Build history of the part. All positions in model axes, mm. Round coordinates to 2 decimals unless told otherwise and drop trailing zeros. Write each loop counter-clockwise with the first axis right and the second up, starting at its lowest first coordinate (ties: lowest second). Pieces come first, ordered by that corner, then holes. Notation, with made-up numbers: (37.25, -34) - (78.25, -34) arc R36 ccw to (78.25, 5) - close; hole circle Ø4 at (59, 35.25). An arc over 180 degrees is marked (long way). Answer as a JSON object with one key per item and string values. Group by question number.
Item 1: Probe line 1 (X direction, y = -0.25, z = 16); line 2 (X direction, y = 0.3, z = 15.25); line 3 (Z direction, x = 4, y = 0.05). List the from-to ranges inside material, lowest first. Write a range as from..to.
Item 2: Slice it at A-A, the plane y = -0.25. List the corners of the cut face in (x, z) (3 decimals).
Item 3: Slice it at D-D, the plane x = 6.75. List the corners of the cut face in (y, z) (3 decimals), then the cut area to 3 significant figures.
Item 4: Slice it at B-B, the plane z = 18.25. List the corners of the cut face in (x, y) (3 decimals), then the cut area to 3 significant figures.
Item 5: Slice it at C-C, the plane x = 10.25. List the corners of the cut face in (y, z) (3 decimals).
Solid Edge part; units mm, degrees
sketch "Sketch1" plane through (0, 0, 0) normal (0, -1, 0) x (1, 0, 0)
  line L0 (0, 0) -> (0, 5.75)
  line L1 (0, 11.5) -> (0, 5.75)
  line L2 (11.625, 21.5) -> (0, 11.5)
  line L3 (14.125, 21.5) -> (11.625, 21.5)
  line L4 (14.125, 21.5) -> (16.625, 21.5)
  line L5 (16.625, 21.5) -> (28.25, 11.5)
  line L6 (28.25, 0) -> (28.25, 11.5)
  line L7 (0, 0) -> (28.25, 0)
  circle A0 centre (14.125, 18.25) radius 0.95
extrude "Protrusion1" add sketch "Sketch1" along normal mid plane 1.25
properties material "Stainless Steel, 420"
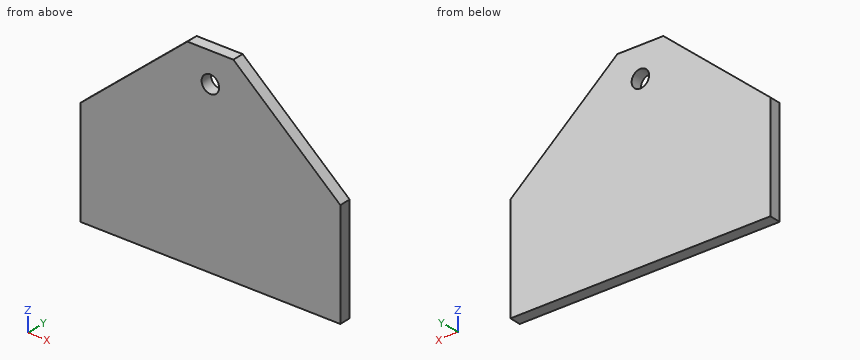
Geometry says:
{
 "1": {"line 1": "x = 5.23..23.02", "line 2": "x = 4.36..23.89", "line 3": "z = 0..14.94"},
 "2": {"outline": "(0, 0) - (28.25, 0) - (28.25, 11.5) - (16.625, 21.5) - (11.625, 21.5) - (0, 11.5) - close; hole circle Ø1.9 at (14.125, 18.25)"},
 "3": {"outline": "(-0.625, 0) - (0.625, 0) - (0.625, 17.306) - (-0.625, 17.306) - close", "area": "21.6 mm^2"},
 "4": {"outline": "(7.847, -0.625) - (13.175, -0.625) - (13.175, 0.625) - (7.847, 0.625) - close; (15.075, -0.625) - (20.403, -0.625) - (20.403, 0.625) - (15.075, 0.625) - close", "area": "13.3 mm^2"},
 "5": {"outline": "(-0.625, 0) - (0.625, 0) - (0.625, 20.317) - (-0.625, 20.317) - close"}
}
